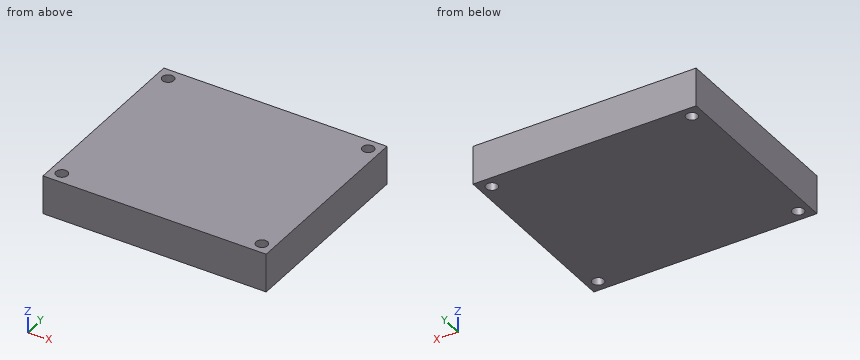
from build123d import *

# Parameters (mm, degrees)
SKETCH_1_W      = 57.849
SKETCH_1_H      = 49.936
SKETCH_1_R      = 1.5
EXTRUDE_1_DEPTH = 10


with BuildPart() as part:
    # 草图1 → 凸台-拉伸1 (new body)
    with BuildSketch(Plane.XY):
        with Locations((25.9245, -21.968)):
            Rectangle(SKETCH_1_W, SKETCH_1_H)
        Circle(SKETCH_1_R, mode=Mode.SUBTRACT)
        with Locations((51.849, 0)):
            Circle(SKETCH_1_R, mode=Mode.SUBTRACT)
        with Locations((51.849, -43.936)):
            Circle(SKETCH_1_R, mode=Mode.SUBTRACT)
        with Locations((0, -43.936)):
            Circle(SKETCH_1_R, mode=Mode.SUBTRACT)
    extrude(amount=EXTRUDE_1_DEPTH)


solid = part.part
For this review, take the finished solid that the model builds, in its own axes (mm). Give positions to 0.01 mm unless a question says otherwise; leave off trailing zeros. Order: outer loops, then holes, each group sorted by start corner. A loop starts at its lowest first (then second) coordinate and runs counter-clockwise, first axis right, second up. Notation, with made-up numbers: (63.5, 52) - (91.5, 52) arc R27 cw to (91.5, 89) - close; hole circle Ø4 at (52, -22.5). An arc over 180 degrees is marked (long way). Answer as a JSON object with one key per item and string values. Group by question number.
Item 1: Take a section at A-A on y = 0. Give the boundary of the cut face in (x, z).
Item 2: Wall thickness on line 1 along Y through (x, z) = (52, 2.5); line 2 along X through (y, z) = (-0.5, 5.75): over which ranges is each line inside the solid? List them lowest first.
Item 3: Take a section at B-B on x = 0. Give the boundary of the cut face in (y, z).
Item 4: Clearance check with a flat-ended pin moving along its axis: pin 1 Ø4 at (x, y) = (0, -43.936) entering from +Z. State where the tip first meets the part, or that it passes through.
Reported:
{
 "1": {"outline": "(-3, 0) - (-1.5, 0) - (-1.5, 10) - (-3, 10) - close; (1.5, 0) - (50.35, 0) - (50.35, 10) - (1.5, 10) - close; (53.35, 0) - (54.85, 0) - (54.85, 10) - (53.35, 10) - close"},
 "2": {"line 1": "-46.94 to -45.43, -42.44 to -1.49, 1.49 to 3", "line 2": "-3 to -1.41, 1.41 to 50.43, 53.26 to 54.85"},
 "3": {"outline": "(-46.94, 0) - (-45.44, 0) - (-45.44, 10) - (-46.94, 10) - close; (-42.44, 0) - (-1.5, 0) - (-1.5, 10) - (-42.44, 10) - close; (1.5, 0) - (3, 0) - (3, 10) - (1.5, 10) - close"},
 "4": {"pin 1": "z = 10"}
}
